The listing builds one solid part. Answer for the finished solid, in the listing's coordinates (mm). A direction names the side the tool comes from. Give positions to 0.01 mm unless a question says otherwise; leave off trailing zeros. Loops run counter-clockwise (first coordinate to the right, second up) from the corner with the lowest first, then second, coordinate; pieces in that order, holes last. Notation, with made-up numbers: M -15.5,-37.75 L 25.5,-37.75 A13 ccw 25.5,-29.75 Z; hole C -5.5,-13 d6. An arc over 180 degrees is marked long. Use one line per item in the form item = value. Start each with the question number.
1. The part is cut by section D-D (x = 24). Write down the section's boundary in (y, z).
2. Straight lines are drawn through the part: line 1 (Y direction, x = 2, z = -27); line 2 (X direction, y = 1.5, z = -22.5); line 3 (X direction, y = 12, z = -1). For each, find the intervals that lie inside material, in ascending order. Write a range as from..to.
3. The part is cut by section C-C (y = 12.25). Write down the section's boundary in (x, z), and give its area (3 significant figures).
4. The part is cut by section A-A (z = 0). Write down the section's boundary in (x, y).
5. For faces 1 (the face through (0, 19, 0)), 2 (the face through (0, 12, -2)), determine the directions among +Z, -Z, +X, -X, +Y, -Y from which every point of the face is accessible in a straight line to the end or side of a thin tool.
6. Each of these flat-tipped pins is pushed along its axis until it touches: pin 1 Ø3 at (y, z) = (6, 17.5) entering from -X; pin 2 Ø6 at (x, y) = (-1, 15.5) entering from +Z; pin 3 Ø4 at (x, y) = (12, 4.5) entering from +Z; pin 4 Ø4 at (x, y) = (-1.5, 5.5) entering from -Z. Where does it stop, or does it pass through?
7. The part is cut by section B-B (x = 0). Write down the section's boundary in (y, z).
from build123d import *

# Parameters (mm, degrees)
CHANFREIN1_SIZE = 1
CHANFREIN2_SIZE = 0.5


with BuildPart() as part:
    # Esquisse1 → Révolution1 (revolve)
    with BuildSketch(Plane.XY):
        Polygon((0, 0), (-30, 0), (-30, 4), (-2, 4), (-2, 19), (0, 19), align=None)
    revolve(axis=Axis((0, 0, 0), (0, 1, 0)))

    # Chanfrein1
    chanfrein1_edges = [part.edges().sort_by_distance(p)[0] for p in [
        (2, 4, 0),
    ]]
    chamfer(chanfrein1_edges, length=CHANFREIN1_SIZE)

    # Chanfrein2
    chanfrein2_edges = [part.edges().sort_by_distance(p)[0] for p in [
        (2, 19, 0),
    ]]
    chamfer(chanfrein2_edges, length=CHANFREIN2_SIZE)


solid = part.part
Derived:
q1.outline = M 0,-18 L 4,-18 L 4,18 L 0,18 Z
q2.line_1 = 0..4
q2.line_2 = -19.84..19.84
q2.line_3 = -1.73..1.73
q3.outline = C 0,0 d4
q3.area = 12.6 mm2
q4.outline = M -30,0 L 30,0 L 30,4 L 3,4 L 2,5 L 2,18.5 L 1.5,19 L -1.5,19 L -2,18.5 L -2,5 L -3,4 L -30,4 Z
q5.face_1 = +Z, -Z, +X, -X, +Y
q5.face_2 = +Y
q6.pin_1 = through
q6.pin_2 = 2
q6.pin_3 = 28.26
q6.pin_4 = -30
q7.outline = M 0,-30 L 4,-30 L 4,-3 L 5,-2 L 18.5,-2 L 19,-1.5 L 19,1.5 L 18.5,2 L 5,2 L 4,3 L 4,30 L 0,30 Z
